```python
from build123d import *

# Parameters (mm, degrees)
SKETCH1_R           = 3.81
SKETCH1_W           = 5.08
SKETCH1_H           = 34.754656801
SKETCH1_W_2         = 31.75
SKETCH1_H_2         = 5.08
SKETCH1_R_2         = 2.54
SKETCH1_W_3         = 38.1
BOSS_EXTRUDE1_DEPTH = 5.08


with BuildPart() as part:
    # Sketch1 → Boss-Extrude1 (new body)
    with BuildSketch(Plane.XY):
        with BuildLine():
            ThreePointArc((51.011314264, 16.355277108), (54.603416713, 17.84317466), (56.091314264, 21.435277108))
            Line((56.091314264, 21.435277108), (56.091314264, 36.675277108))
            ThreePointArc((56.091314264, 36.675277108), (57.579211816, 40.267379557), (61.171314264, 41.755277108))
            Line((61.171314264, 41.755277108), (76.411314264, 41.755277108))
            ThreePointArc((76.411314264, 41.755277108), (80.003416713, 43.24317466), (81.491314264, 46.835277108))
            Line((81.491314264, 46.835277108), (81.491314264, 155.588877174))
            ThreePointArc((81.491314264, 155.588877174), (80.003416713, 159.180979622), (76.411314264, 160.668877174))
            Line((76.411314264, 160.668877174), (61.171314264, 160.668877174))
            ThreePointArc((61.171314264, 160.668877174), (57.579211816, 162.156774726), (56.091314264, 165.748877174))
            Line((56.091314264, 165.748877174), (56.091314264, 180.988877174))
            ThreePointArc((56.091314264, 180.988877174), (54.603416713, 184.580979622), (51.011314264, 186.068877174))
            Line((51.011314264, 186.068877174), (-144.469703574, 186.068877174))
            ThreePointArc((-144.469703574, 186.068877174), (-148.061806022, 184.580979622), (-149.549703574, 180.988877174))
            Line((-149.549703574, 180.988877174), (-149.549703574, 165.748877174))
            ThreePointArc((-149.549703574, 165.748877174), (-151.037601126, 162.156774726), (-154.629703574, 160.668877174))
            Line((-154.629703574, 160.668877174), (-169.869703574, 160.668877174))
            ThreePointArc((-169.869703574, 160.668877174), (-173.461806022, 159.180979622), (-174.949703574, 155.588877174))
            Line((-174.949703574, 155.588877174), (-174.949703574, 46.835277108))
            ThreePointArc((-174.949703574, 46.835277108), (-173.461806022, 43.24317466), (-169.869703574, 41.755277108))
            Line((-169.869703574, 41.755277108), (-154.629703574, 41.755277108))
            ThreePointArc((-154.629703574, 41.755277108), (-151.037601126, 40.267379557), (-149.549703574, 36.675277108))
            Line((-149.549703574, 36.675277108), (-149.549703574, 21.435277108))
            ThreePointArc((-149.549703574, 21.435277108), (-148.061806022, 17.84317466), (-144.469703574, 16.355277108))
            Line((-144.469703574, 16.355277108), (51.011314264, 16.355277108))
        make_face()
        with Locations((-110.682245407, 29.055277108)):
            Circle(SKETCH1_R, mode=Mode.SUBTRACT)
        Polygon((-25.922239135, 55.997635261), (-25.922239135, 49.700309173), (-25.922239135, 46.781251801), (-86.372159657, 46.781251801), (-86.372159657, 55.997635261), align=None, mode=Mode.SUBTRACT)
        with Locations((-162.249703574, 70.149378101)):
            Circle(SKETCH1_R, mode=Mode.SUBTRACT)
        Polygon((-25.922239135, 84.197043075), (-25.922239135, 77.899716987), (-25.922239135, 74.980659615), (-86.372159657, 74.980659615), (-86.372159657, 84.197043075), (-62.604194655, 84.197043075), (-62.604194655, 90.255887093), (-30.854194655, 90.255887093), (-30.854194655, 84.197043075), align=None, mode=Mode.SUBTRACT)
        with Locations((17.223856098, 29.055277108)):
            Circle(SKETCH1_R, mode=Mode.SUBTRACT)
        with Locations((0.772267685, 66.819714675)):
            Rectangle(SKETCH1_W, SKETCH1_H, mode=Mode.SUBTRACT)
        with Locations((-46.729194655, 97.608815198)):
            Rectangle(SKETCH1_W_2, SKETCH1_H_2, mode=Mode.SUBTRACT)
        with Locations((68.791314264, 70.149378101)):
            Circle(SKETCH1_R, mode=Mode.SUBTRACT)
        Polygon((-149.549703574, 135.965208253), (-144.469703574, 135.965208253), (-144.469703574, 127.195635913), (-144.469703574, 102.945208253), (-149.549703574, 102.945208253), align=None, mode=Mode.SUBTRACT)
        with Locations((-137.903692136, 121.995208253)):
            Circle(SKETCH1_R_2, mode=Mode.SUBTRACT)
        with Locations((-162.249703574, 132.274776181)):
            Circle(SKETCH1_R, mode=Mode.SUBTRACT)
        with Locations((-91.632245407, 102.945208253)):
            Circle(SKETCH1_R_2, mode=Mode.SUBTRACT)
        with Locations((-110.682245407, 141.140921067)):
            Rectangle(SKETCH1_W_3, SKETCH1_H_2, mode=Mode.SUBTRACT)
        with Locations((-110.682245407, 173.368877174)):
            Circle(SKETCH1_R, mode=Mode.SUBTRACT)
        with Locations((-46.729194655, 108.841683137)):
            Rectangle(SKETCH1_W_2, SKETCH1_H_2, mode=Mode.SUBTRACT)
        with Locations((-1.826143902, 102.945208253)):
            Circle(SKETCH1_R_2, mode=Mode.SUBTRACT)
        with BuildLine():
            ThreePointArc((33.767746549, 132.274776181), (35.563797773, 131.530827406), (36.307746549, 129.734776181))
            Line((36.307746549, 129.734776181), (36.307746549, 127.195635913))
            Line((36.307746549, 127.195635913), (36.307746549, 116.226694176))
            ThreePointArc((36.307746549, 116.226694176), (35.563797773, 114.430642952), (33.767746549, 113.686694176))
            Line((33.767746549, 113.686694176), (-127.226135859, 113.686694176))
            ThreePointArc((-127.226135859, 113.686694176), (-129.022187083, 114.430642952), (-129.766135859, 116.226694176))
            Line((-129.766135859, 116.226694176), (-129.766135859, 127.195635913))
            Line((-129.766135859, 127.195635913), (-129.766135859, 129.734776181))
            ThreePointArc((-129.766135859, 129.734776181), (-129.022187083, 131.530827406), (-127.226135859, 132.274776181))
            Line((-127.226135859, 132.274776181), (33.767746549, 132.274776181))
        make_face(mode=Mode.SUBTRACT)
        with Locations((-46.729194655, 138.978682913)):
            Rectangle(SKETCH1_W_2, SKETCH1_H_2, mode=Mode.SUBTRACT)
        with Locations((17.223856098, 141.140921067)):
            Rectangle(SKETCH1_W_3, SKETCH1_H_2, mode=Mode.SUBTRACT)
        with Locations((44.445302826, 121.995208253)):
            Circle(SKETCH1_R_2, mode=Mode.SUBTRACT)
        Polygon((51.011314264, 127.195635913), (51.011314264, 135.965208253), (56.091314264, 135.965208253), (56.091314264, 102.945208253), (51.011314264, 102.945208253), align=None, mode=Mode.SUBTRACT)
        with Locations((68.791314264, 132.274776181)):
            Circle(SKETCH1_R, mode=Mode.SUBTRACT)
        with Locations((-46.729194655, 150.112295085)):
            Rectangle(SKETCH1_W_2, SKETCH1_H_2, mode=Mode.SUBTRACT)
        with Locations((17.223856098, 173.368877174)):
            Circle(SKETCH1_R, mode=Mode.SUBTRACT)
    extrude(amount=BOSS_EXTRUDE1_DEPTH)


solid = part.part
```
Work out the finished part from the listing and answer in its coordinate system (mm). A direction names the side the tool comes from. Give positions to 0.01 mm unless a question says otherwise; leave off trailing zeros. Answer as CSV lines item,"result". Start each with the question number.
(1) Which of the six approach directions +Z, -Z, +X, -X, +Y, -Y give full straight-line access (tool end or side, diameter ignored) to faces 1 (the flat face through (69, 41.755, 3)), 2 (the flat face through (-111, 143.681, 3))?
(2) Consider line 1 along Y through (x, z) = (-98.5, 3.6); line 2 along Y through (x, z) = (-26, 1.6); line 3 along Y through (x, z) = (17, 0.65). Determine where each line is inside the solid, lowest interval first.
(3) Section A-A, the plane x = -44.5 is taken. Give the number of separate pieces and of enclosed holes in the cut face, plus the area to 3 significant figures.
(4) Each of these flat-tipped pins is pushed along its axis until it touches: pin 1 Ø1.5 at (x, z) = (52.5, 3) entering from +Y; pin 2 Ø4.5 at (x, y) = (-110.68, 173.37) entering from -Z. Where does it stop, or does it pass through?
(5) For a pull along X with two mould halves and no side action, classify faces 3 (the flat face through (-174.95, 102, 3)), 4 (the flat face through (17, 138.601, 3)), 5 (the cylindrical face through (54.56, 17.8, 2.5)) as released by +X, released by -X, zero draft, split by the parting line, or undercut.
Entries:
1,face 1,"+Z, -Z, +X, -Y"
1,face 2,"+Z, -Z"
2,line 1,"16.36 to 113.69, 132.27 to 138.6, 143.68 to 186.07"
2,line 2,"16.36 to 46.78, 56 to 74.98, 84.2 to 113.69, 132.27 to 186.07"
2,line 3,"16.36 to 25.25, 32.86 to 113.69, 132.27 to 138.6, 143.68 to 169.57, 177.17 to 186.07"
3,separate pieces,"8"
3,enclosed holes,"0"
3,area,"540 mm²"
4,pin 1,"y = 186.01"
4,pin 2,"through"
5,face 3,"released by -X"
5,face 4,"undercut"
5,face 5,"released by +X"
